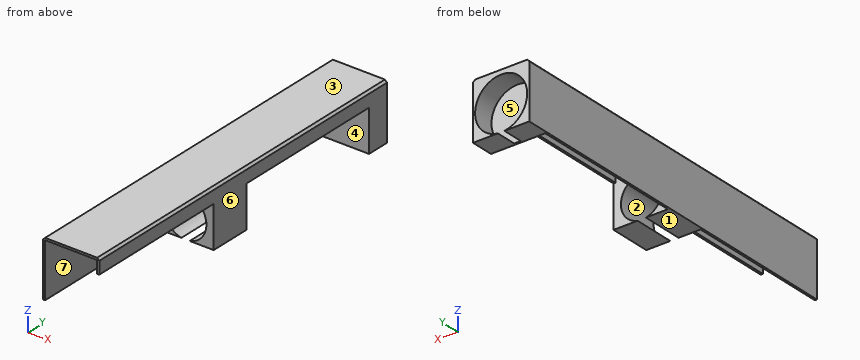
```python
from build123d import *

# Parameters (mm, degrees)
F1_DEPTH  = 176
F3_W      = 25
F3_H      = 1
F4_DEPTH  = 26
F5_DEPTH  = 10
F6_R      = 12.5
F7_DEPTH  = 10
F8_W      = 75
F8_H      = 20
F8_W_2    = 70
F9_DEPTH  = 1
F10_W     = 25
F10_H     = 20
F11_DEPTH = 26
F12_R     = 10
F13_DEPTH = 20
F14_SIZE  = 1


with BuildPart() as f1:
    # F0 (on Front) → F1 (new body)
    with BuildSketch(Plane.XZ):
        Polygon((0, 27), (0, 0), (1, 0), (1, 26), (13.5, 26), (13.5, 27), align=None)
    extrude(amount=F1_DEPTH)

    # F2: F1 across face


with BuildPart() as f1_1:
    add(f1.part)
    add(f1.part.mirror(Plane(origin=(13.5, -88, 26.5), x_dir=(0, 1, 0), z_dir=(1, 0, 0))))

    # F3 (on face) → F4 (join)
    with BuildSketch(Plane(origin=(0, 0, 26), x_dir=(1, 0, 0), z_dir=(0, 0, -1))):
        with Locations((13.5, 10.5)):
            Rectangle(F3_W, F3_H)
    extrude(amount=F4_DEPTH)

    # F5 (add, through all): a face of the model
    f5_faces = [f1_1.faces().sort_by_distance(p)[0] for p in [
        (13.5, -10, 13),
    ]]
    extrude(f5_faces, amount=F5_DEPTH)

    # F6 (on face) → F7 (cut)
    with BuildSketch(Plane(origin=(0, 0, 0), x_dir=(-1, 0, 0), z_dir=(0, 1, 0))):
        with Locations((-13.5, 12.4)):
            Circle(F6_R)
    extrude(amount=-F7_DEPTH, mode=Mode.SUBTRACT)

    # F8 (on face) → F9 (cut, through all)
    with BuildSketch(Plane.YZ.offset(27)):
        with Locations((-48.5, 10)):
            Rectangle(F8_W, F8_H)
        with Locations((-141, 10)):
            Rectangle(F8_W_2, F8_H)
    extrude(amount=-F9_DEPTH, mode=Mode.SUBTRACT)

    # F10 (on face) → F11 (join, through all)
    with BuildSketch(Plane(origin=(0, 0, 26), x_dir=(1, 0, 0), z_dir=(0, 0, -1))):
        with Locations((13.5, 96)):
            Rectangle(F10_W, F10_H)
    extrude(amount=F11_DEPTH)

    # F12 (on face) → F13 (cut, through all)
    with BuildSketch(Plane.XZ.offset(106)):
        with Locations((13.5, 9.8)):
            Circle(F12_R)
    extrude(amount=-F13_DEPTH, mode=Mode.SUBTRACT)

    # F14
    f14_edges = [f1_1.edges().sort_by_distance(p)[0] for p in [
        (27, -88, 27),
        (0, -88, 27),
    ]]
    chamfer(f14_edges, length=F14_SIZE)


solid = f1_1.part
```
Here's how the part is built. I have some questions about the finished solid (model axes, mm). Face numbers are marked on the shaded views. A direction names the side the tool comes from. Coordinates: 2 decimals unless noted, no trailing zeros. Write each loop counter-clockwise with the first axis right and the second up, starting at its lowest first coordinate (ties: lowest second). Pieces come first, ordered by that corner, then holes. Notation, with made-up numbers: (0, 8.5) - (19, 8.5) arc R23 cw to (19, 41.5) - close; hole circle Ø4 at (-15.75, -21.75). An arc over 180 degrees is marked (long way). One line per item, written item: value.
1) On a 3-axis mill with a long thin cutter (end or side, diameter ignored), from which of +Z, -Z, +X, -X, +Y, -Y can I reach the whole of each face in a straight line? I mean the marked faces 4, 5, 6 and 7. Say none if no direction works.
Model answer:
face 4: -Z
face 5: +Y
face 6: +Z, -Z, +X, +Y, -Y
face 7: -Z, -Y
2) We'd pull the mould along Z, two halves only. Please class the marked faces 1, 2 and 3: pulls with the +Z half, pulls with the -Z half, needs draft (parallel to the pull), parting line crosses it, or undercut.
Model answer:
face 1: pulls with the -Z half
face 2: undercut
face 3: pulls with the +Z half
3) Suppose I cut it at A-A on x = 7.25. Write out the boundary of the cut face in (y, z), and give its area (3 significant figures).
Model answer:
outline: (-176, 26) - (-106, 26) - (-106, 17.61) - (-86, 17.61) - (-86, 26) - (-11, 26) - (-11, 0) - (0, 0) - (0, 1.57) - (-10, 1.57) - (-10, 23.23) - (0, 23.23) - (0, 27) - (-176, 27) - close; (-106, 0) - (-86, 0) - (-86, 1.99) - (-106, 1.99) - close
area: 453 mm²
4) Suppose I cut it at D-D on z = 22.5. Write out the boundary of the cut face in (x, y), and give its area (3 significant figures).
Model answer:
outline: (0, -176) - (1, -176) - (1, -106) - (26, -106) - (26, -176) - (27, -176) - (27, 0) - (20.86, 0) - (20.86, -10) - (6.14, -10) - (6.14, 0) - (0, 0) - close; hole (1, -86) - (26, -86) - (26, -11) - (1, -11) - close
area: 980 mm²
5) Suppose I cut it at C-C on y = -109. Write out the boundary of the cut face in (x, z).
Model answer:
outline: (0, 0) - (1, 0) - (1, 26) - (26, 26) - (26, 20) - (27, 20) - (27, 26) - (26, 27) - (1, 27) - (0, 26) - close
6) Suppose I cut it at B-B on z = 4.5. Write out the boundary of the cut face in (x, y).
Model answer:
outline: (0, -176) - (1, -176) - (1, -106) - (5.02, -106) - (5.02, -86) - (1, -86) - (1, -11) - (27, -11) - (27, 0) - (23.19, 0) - (23.19, -10) - (3.81, -10) - (3.81, 0) - (0, 0) - close; (21.98, -106) - (27, -106) - (27, -86) - (21.98, -86) - close
7) I'm going to push flat-ended pins straight in: P1, Ø13, axis at y = -35.5, z = 10, coming from the +X side; P2, Ø8, axis at x = 17, z = 13, coming from the +Y side; P3, Ø2, axis at x = 5.5, z = 5, coming from the -Y side. Where does each tip first touch, or does it pass through?
Model answer:
P1: stops at x = 1
P2: stops at y = -10
P3: stops at y = -106
8) I need wall thicknesses on line 1 along Y through (x, z) = (1.75, 9.75); line 2 along X through (y, z) = (-94, 9.8); line 3 along X through (y, z) = (-5.5, 12.4). Which ranges of each line are inside material? Lowest first, please.
Model answer:
line 1: y = -106 to -86, -11 to -10
line 2: x = 0 to 3.5, 23.5 to 27
line 3: x = 0 to 1, 26 to 27
